The drawing under review shows one solid part. Ordinate dimensions are in mm from its lowest x, y, z. Give positions to 0.01 mm unless a question says otherwise; leave off trailing zeros. Order: outer loops, then holes, each group sorted by start corner. A loop starts at its lowest first (then second) coordinate and runs counter-clockwise, first axis right, second up. Notation, with made-up numbers: (10.25, 42) -> (49.25, 42) arc R20 cw to (49.25, 68) -> close; hole circle Ø7 at (83, 26). An arc over 180 degrees is marked (long way). Return JSON: item names as keys, results as strings. Group by question number.
1) To check wall thickness, follow line 1 along Y through (x, z) = (2.55, 12.7); line 2 along Z through (x, y) = (14.75, 252) (1 decimal); line 3 along Y through (x, z) = (12.7, 23.35). State the ranges of each line that lie inside material, in increasing order.
2) Insertion check: P1, Ø1.5, axis at x = 11, y = 246, coming from the -Z side. The pin has a flat end and moves straight along its axis. Give the tip position at first contact, or say it passes through.
3) Add section B-B (z = 12.7). Give the boundary of the cut face in (x, y) (1 decimal).
4) Add section A-A (x = 6.25). Give the boundary of the cut face in (y, z) (1 decimal), then the cut area to 3 significant figures.
5) Add section C-C (y = 323.5). Give the boundary of the cut face in (x, z) (1 decimal).
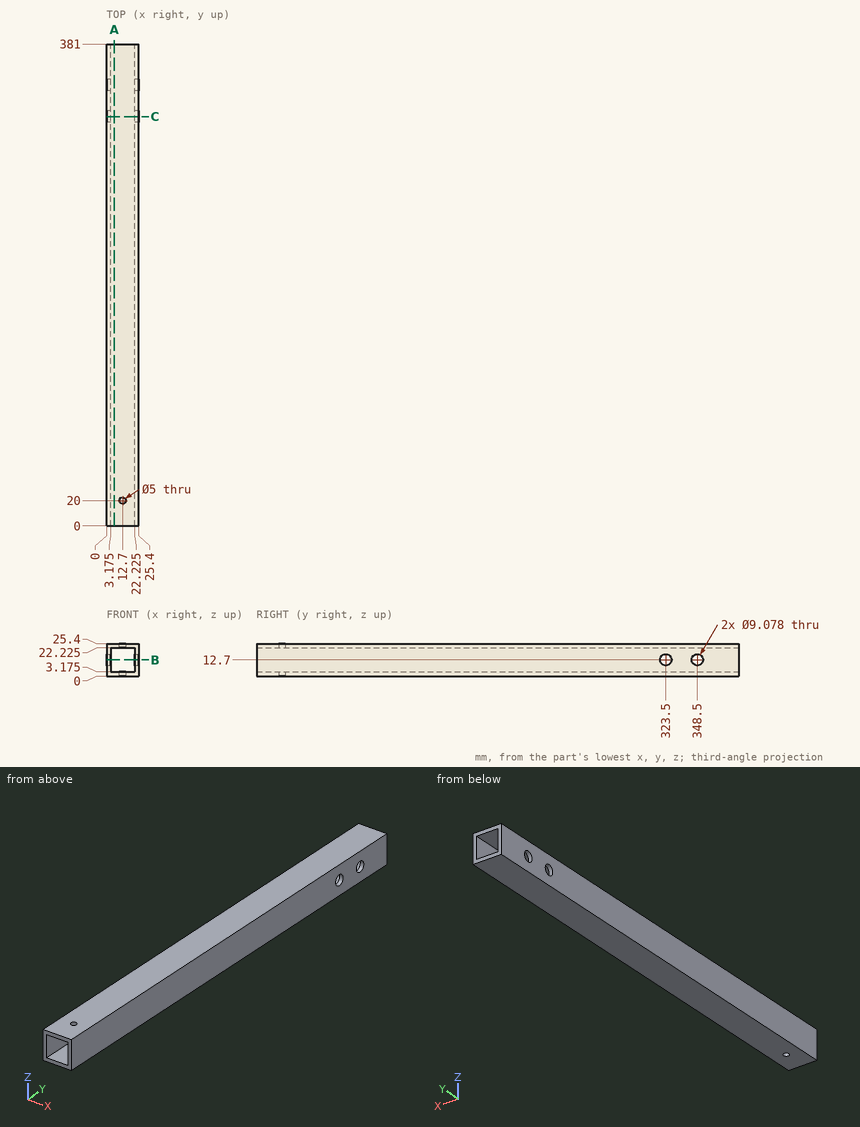
Evaluation:
{
 "1": {"line 1": "0 to 318.96, 328.04 to 343.96, 353.04 to 381", "line 2": "0 to 3.2, 22.2 to 25.4", "line 3": "0 to 17.5, 22.5 to 381"},
 "2": {"P1": "z = 0"},
 "3": {"outline": "(0, 0) -> (3.2, 0) -> (3.2, 319) -> (0, 319) -> close; (0, 328) -> (3.2, 328) -> (3.2, 344) -> (0, 344) -> close; (0, 353) -> (3.2, 353) -> (3.2, 381) -> (0, 381) -> close; (22.2, 0) -> (25.4, 0) -> (25.4, 319) -> (22.2, 319) -> close; (22.2, 328) -> (25.4, 328) -> (25.4, 344) -> (22.2, 344) -> close; (22.2, 353) -> (25.4, 353) -> (25.4, 381) -> (22.2, 381) -> close"},
 "4": {"outline": "(0, 0) -> (381, 0) -> (381, 3.2) -> (0, 3.2) -> close; (0, 22.2) -> (381, 22.2) -> (381, 25.4) -> (0, 25.4) -> close", "area": "2,420 mm^2"},
 "5": {"outline": "(0, 0) -> (25.4, 0) -> (25.4, 8.2) -> (22.2, 8.2) -> (22.2, 3.2) -> (3.2, 3.2) -> (3.2, 8.2) -> (0, 8.2) -> close; (0, 17.2) -> (3.2, 17.2) -> (3.2, 22.2) -> (22.2, 22.2) -> (22.2, 17.2) -> (25.4, 17.2) -> (25.4, 25.4) -> (0, 25.4) -> close"}
}
